from build123d import *

# Parameters (mm, degrees)
F1_DEPTH = 63.5
F0_W     = 25.4
F0_H     = 19.05
F2_DEPTH = 25.4
F3_DEPTH = 12.7
F6_D     = 25.4


with BuildPart() as f1:
    # F0 (on Front) → F1 (new body, symmetric)
    with BuildSketch(Plane.XZ):
        Polygon((41.275, -9.525), (41.275, 9.525), (22.225, 9.525), (-41.275, 9.525), (-41.275, -9.525), align=None)
    extrude(amount=F1_DEPTH, both=True)

    # F0 (on Front) → F2 (join, symmetric)
    with BuildSketch(Plane.XZ):
        with BuildLine():
            Line((22.225, 9.525), (41.275, 9.525))
            Line((41.275, 9.525), (41.275, 27.0002))
            ThreePointArc((41.275, 27.0002), (45.9246798487, 38.2255201513), (57.15, 42.8752))
            Line((57.15, 42.8752), (60.325, 42.8752))
            Line((60.325, 42.8752), (60.325, 61.9252))
            Line((60.325, 61.9252), (57.15, 61.9252))
            ThreePointArc((57.15, 61.9252), (32.4542956671, 51.6959043329), (22.225, 27.0002))
            Line((22.225, 27.0002), (22.225, 9.525))
        make_face()
        with Locations((73.025, 52.4002)):
            Rectangle(F0_W, F0_H)
    extrude(amount=F2_DEPTH, both=True)

    # F0 (on Front) → F3 (join, symmetric)
    with BuildSketch(Plane.XZ):
        with BuildLine():
            Line((-41.275, 9.525), (22.225, 9.525))
            Line((22.225, 9.525), (22.225, 27.0002))
            ThreePointArc((22.225, 27.0002), (32.4542956671, 51.6959043329), (57.15, 61.9252))
            add(Edge.make_bspline(
                [(57.15, 61.9252), (2.3303949274, 65.2119144797), (-40.8146418631, 33.2797057927), (-41.275, 9.525)],
                knots=[0, 0, 0, 0, 111.5045361635, 111.5045361635, 111.5045361635, 111.5045361635], degree=3))
        make_face()
    extrude(amount=F3_DEPTH, both=True)

    # F0 (on Front) → F4 (revolve)
    with BuildSketch(Plane.XZ):
        Polygon((85.725, 61.9252), (85.725, 42.8752), (85.725, 38.1), (111.125, 38.1), (111.125, 66.675), (85.725, 66.675), align=None)
    revolve(axis=Axis((85.725, 0, 52.3875), (0, 0, -1)))

    # F6 (through all)
    with Locations(Plane.XY.offset(66.675)):
        with Locations((85.725, 0)):
            Hole(F6_D / 2)


solid = f1.part
Work out the finished part from the listing and answer in its coordinate system (mm). A direction names the side the tool comes from. Round coordinates to 2 decimals unless told otherwise and drop trailing zeros. Loops run counter-clockwise (first coordinate to the right, second up) from the corner with the lowest first, then second, coordinate; pieces in that order, holes last. Notation, with made-up numbers: (44, 40.5) -> (72, 40.5) arc R24 cw to (72, 58.5) -> close; hole circle Ø4 at (76.25, 8). An arc over 180 degrees is marked (long way). Use one line per item in the form item = value.
(1) Find section A-A on y = 37. Give the vertices of the cut face in (x, z) (3 decimals).
Answer list:
outline = (-41.275, -9.525) -> (41.275, -9.525) -> (41.275, 9.525) -> (-41.275, 9.525) -> close
(2) Flat-ended cylindrical pins translate along their axes: P1, Ø14, axis at y = 20, z = 18, coming from the -X side (3 decimals); P2, Ø2, axis at y = 23, z = 25, coming from the +X side (3 decimals); P3, Ø23, axis at x = 71, y = 4.5, coming from the -Z side; P4, Ø8.5, axis at x = 76.5, y = 6, coming from the +Z side (3 decimals). Find the tip coordinate at first contact, or state that the pin passes through.
Answer list:
P1 = 22.225
P2 = 41.275
P3 = 38.1
P4 = 66.675
(3) For a pull along X with two mould halves and no side action, classify faces 6 (the cylindrical face through (45.8, -0.4, 38.1)), 7 (the flat face through (60, -2, 61.925)), 8 (the flat face through (-41.275, -1, 0)), 9 (the flat face through (41.275, -1, 4)) as released by +X, released by -X, zero draft, split by the parting line, or undercut.
Answer list:
face_6 = undercut
face_7 = undercut
face_8 = released by -X
face_9 = released by +X
(4) Straight lines are drawn through the part: line 1 (X direction, y = -17, z = 24.5) (3 decimals); line 2 (X direction, y = -38.5, z = 1) (3 decimals); line 3 (Y direction, x = 28, z = 52.5). For each, find the intervals that lie inside material, in ascending order.
Answer list:
line_1 = 22.225 to 41.275
line_2 = -41.275 to 41.275
line_3 = -12.7 to 12.7
(5) A tool of negligible diameter and unlimited length cuts with its end or side. For faces 1 (the flat face through (46, -25.4, 42)), 2 (the flat face through (80, -12, 38.1)), 3 (the flat face through (-1, -1, -9.525)), 4 (the cylindrical face through (32.73, -19.14, 51.97)), 5 (the cylindrical face through (32.73, 18.96, 51.97)), from which of +Z, -Z, +X, -X, +Y, -Y can it reach the whole face along a straight path? Write none if from no direction.
Answer list:
face_1 = +Z, +X, -X, -Y
face_2 = -Z, +X, +Y, -Y
face_3 = -Z, +X, -X, +Y, -Y
face_4 = +Z, -X, -Y
face_5 = +Z, -X, +Y
